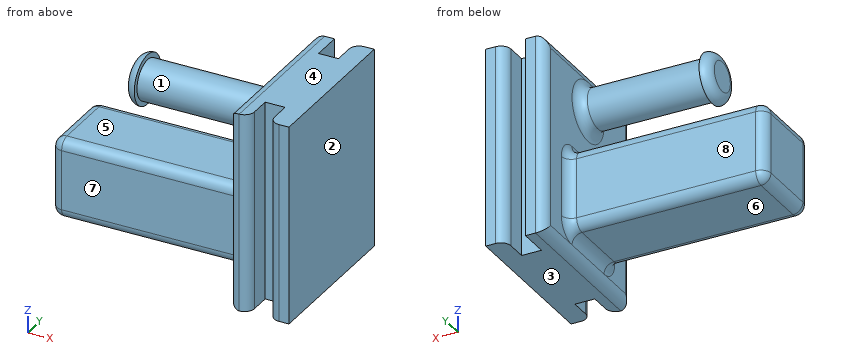
from build123d import *

# Parameters (mm, degrees)
SKETCH1_W           = 2
SKETCH1_H           = 10
BOSS_EXTRUDE1_DEPTH = 20
SKETCH2_R           = 2
BOSS_EXTRUDE2_DEPTH = 13.5
SKETCH3_R           = 2.5
BOSS_EXTRUDE3_DEPTH = 1
SKETCH4_W           = 8
SKETCH4_H           = 8
BOSS_EXTRUDE4_DEPTH = 20
FILLET1_R           = 1


with BuildPart() as part:
    # Sketch1 → Boss-Extrude1 (new body)
    with BuildSketch(Plane.XY):
        Polygon((-1, -8), (-1, -5), (-1, 5), (-1, 8), (-3, 8), (-3, -8), align=None)
        Rectangle(SKETCH1_W, SKETCH1_H)
        Polygon((1, 5), (1, -5), (1, -8), (3, -8), (3, 8), (1, 8), align=None)
    extrude(amount=BOSS_EXTRUDE1_DEPTH)

    # Sketch2 → Boss-Extrude2 (add)
    with BuildSketch(Plane.ZY.offset(3)):
        with Locations((16, 0)):
            Circle(SKETCH2_R)
    extrude(amount=BOSS_EXTRUDE2_DEPTH)

    # Sketch3 → Boss-Extrude3 (add)
    with BuildSketch(Plane.ZY.offset(16.5)):
        with Locations((16, 0)):
            Circle(SKETCH3_R)
    extrude(amount=-BOSS_EXTRUDE3_DEPTH)

    # Sketch4 → Boss-Extrude4 (add)
    with BuildSketch(Plane.ZY.offset(3)):
        with Locations((6, 0)):
            Rectangle(SKETCH4_W, SKETCH4_H)
    extrude(amount=BOSS_EXTRUDE4_DEPTH)

    # Fillet1
    fillet1_edges = [part.edges().sort_by_distance(p)[0] for p in [
        (-3, 0, 0),
        (-3, -8, 10),
        (-3, 8, 10),
        (1, 8, 10),
        (1, -8, 10),
        (-1, -8, 10),
        (-3, 0, 14),
        (-16.5, 0, 13.5),
        (-3, 0, 20),
        (-3, 0, 10),
        (-13, -4, 10),
        (-3, 4, 6),
        (-13, 4, 10),
        (-3, 0, 2),
        (-13, 4, 2),
        (-3, -4, 6),
        (-13, -4, 2),
        (-23, 0, 10),
        (-23, 4, 6),
        (-23, 0, 2),
        (-23, -4, 6),
    ]]
    fillet(fillet1_edges, radius=FILLET1_R - 0.0001)  # a hair under: the kernel refuses the full size


solid = part.part
Source: CAD feature listing. Evaluate the final solid. Frame: model axes, mm. Face numbers are marked on the shaded views. A direction names the side the tool comes from. Round coordinates to 2 decimals unless told otherwise and drop trailing zeros. Loops run counter-clockwise (first coordinate to the right, second up) from the corner with the lowest first, then second, coordinate; pieces in that order, holes last. Notation, with made-up numbers: M -12.5,-34.5 L 3.5,-34.5 A15 cw 3.5,-8.5 Z; hole C 67,-7 d7. An arc over 180 degrees is marked long. Return JSON: item names as keys, results as strings. Group by question number.
1. Section query A-A on x = -11.75. Output: boundary loops of the cut face in (y, z), and give its area (3 significant figures).
2. Pin query (flat end, axial travel): pin 1 (6.5 mm diameter, centred on x = -15, y = 1, fed in from -Z); pin 2 (1.6 mm diameter, centred on x = 0, z = 8, fed in from +Y); pin 3 (3.5 mm diameter, centred on y = -0.5, z = 16.5, fed in from -X). Return the tip coordinate at first contact, or that it passes through.
3. Reachability of the marked faces 4, 5, 6, 7 and 8 from +Z, -Z, +X, -X, +Y, -Y: full face, straight path, thin tool, end or side. Return the list, or none.
4. Section query B-B on y = -6.25. Output: boundary loops of the cut face in (x, z).
5. Mould query, pull axis X, two halves, no side actions, for the marked faces 1, 2 and 3. Classes: released by +X, released by -X, zero draft, split by the parting line, or undercut.
6. Material intervals for line 1 along X through (y, z) = (5.25, 10.25); line 2 along X through (y, z) = (-3.25, 18.25); line 3 along Z through (x, y) = (-5.75, 0.5), sorted ascending. Write a range as from..to.
Checks:
{
 "1": {"outline": "M -4,3 A1 ccw -3,2 L 3,2 A1 ccw 4,3 L 4,9 A1 ccw 3,10 L -3,10 A1 ccw -4,9 Z; C 0,16 d4", "area": "75.7 mm²"},
 "2": {"pin 1": "stops at z = 2", "pin 2": "stops at y = 5", "pin 3": "stops at x = -16.5"},
 "3": {"face 4": "+Z, +X, -X, +Y, -Y", "face 5": "-X, +Y, -Y", "face 6": "-Z, -X, +Y, -Y", "face 7": "+Z, -Z, -X, -Y", "face 8": "+Z, -Z, -X, +Y"},
 "4": {"outline": "M -3,1 A1 ccw -2,0 L -1,0 L -1,20 L -2,20 A1 ccw -3,19 Z; M 1,0 L 3,0 L 3,20 L 1,20 Z"},
 "5": {"face 1": "undercut", "face 2": "released by +X", "face 3": "zero draft"},
 "6": {"line 1": "x = -3..-1, 1..3", "line 2": "x = -3..3", "line 3": "z = 2..10, 14.06..17.94"}
}
